Geometry check sheet. Reference: drawing and pictorial views, mm from the part's lowest x, y, z. Give positions to 0.01 mm unless a question says otherwise; leave off trailing zeros. Write each loop counter-clockwise with the first axis right and the second up, starting at its lowest first coordinate (ties: lowest second). Pieces come first, ordered by that corner, then holes. Notation, with made-up numbers: (-38, 59.25) - (5, 59.25) arc R35 cw to (5, 95.25) - close; hole circle Ø6 at (84.25, 80). An arc over 180 degrees is marked (long way). Put each result on its own line as item: value.
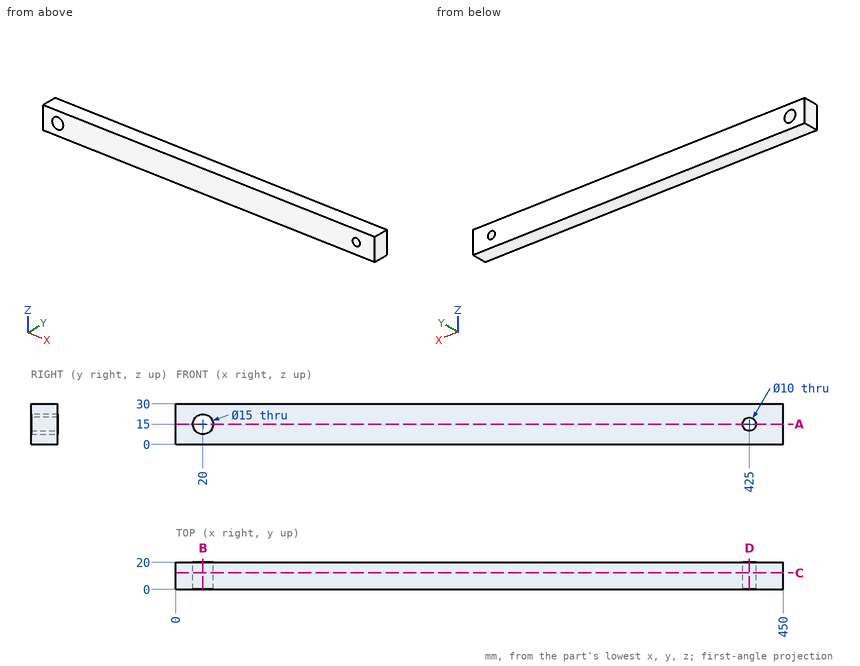
Q1. Section check A-A, the plane z = 15. Record the cut outline in (x, y), plus the area to 3 significant figures.
Answers follow:
outline: (0, 0) - (12.5, 0) - (12.5, 20) - (0, 20) - close; (27.5, 0) - (420, 0) - (420, 20) - (27.5, 20) - close; (430, 0) - (450, 0) - (450, 20) - (430, 20) - close
area: 8,500 mm2
Q2. Section check D-D, the plane x = 425. Record the cut outline in (y, z).
Answers follow:
outline: (0, 0) - (20, 0) - (20, 10) - (0, 10) - close; (0, 20) - (20, 20) - (20, 30) - (0, 30) - close
Q3. Section check C-C, the plane y = 12.25. Record the cut outline in (x, z).
Answers follow:
outline: (0, 0) - (450, 0) - (450, 30) - (0, 30) - close; hole circle Ø15 at (20, 15); hole circle Ø10 at (425, 15)
Q4. Scan lines: line 1 along X through (y, z) = (1.25, 14.5); line 2 along Z through (x, y) = (425, 6); line 3 along X through (y, z) = (7.5, 15.75). Record each from-to range of solid material in increasing order.
Answers follow:
line 1: x = 0 to 12.52, 27.48 to 420.03, 429.97 to 450
line 2: z = 0 to 10, 20 to 30
line 3: x = 0 to 12.54, 27.46 to 420.06, 429.94 to 450
Q5. Section check B-B, the plane x = 20. Record the cut outline in (y, z).
Answers follow:
outline: (0, 0) - (20, 0) - (20, 7.5) - (0, 7.5) - close; (0, 22.5) - (20, 22.5) - (20, 30) - (0, 30) - close
Q6. Go/stop test with a flat-tipped pin: pin 1 Ø4 at (y, z) = (10, 4) entering from -X. Record where the tip stops, or that it passes through.
Answers follow:
pin 1: stops at x = 0
